Read the model definition and answer for the solid it produces. Units are mm, in the model's axes. Face numbers are marked on the shaded views. Coordinates: 2 decimals unless noted, no trailing zeros. Order: outer loops, then holes, each group sorted by start corner. A loop starts at its lowest first (then second) coordinate and runs counter-clockwise, first axis right, second up. Notation, with made-up numbers: (12, -2.5) - (69, -2.5) arc R13 ccw to (69, 21.5) - close; hole circle Ø2 at (-5.75, 83). An arc over 180 degrees is marked (long way). Write item = value, one per line.
from build123d import *

# Parameters (mm, degrees)
EXTRUDE_START       = -10
SKETCH_1_R          = 3.5
EXTRUDE_1_DEPTH     = 85
SKETCH_2_W          = 4.358557255
SKETCH_2_H          = 19.447665258
SKETCH_2_W_2        = 4.358557256
CUT_EXTRUDE_2_DEPTH = 9
SKETCH_3_R          = 1
CUT_EXTRUDE_3_DEPTH = 9


with BuildPart() as part:
    # Эскиз1 → Вытянуть1 (new body)
    with BuildSketch(Plane(origin=(0, 0, 0), x_dir=(1, 0, 0), z_dir=(0, 1, 0)).offset(EXTRUDE_START)):
        with Locations(Location((1.708090692, -2.563541488, 0), (0, 0, 270))):
            Circle(SKETCH_1_R)
    extrude(amount=EXTRUDE_1_DEPTH)

    # Эскиз2 → Вытянуть2 (cut, symmetric)
    with BuildSketch(Plane(origin=(0, 0, 0), x_dir=(0, 0, -1), z_dir=(1, 0, 0))):
        with Locations((-7.693664616, 8.043574294)):
            Rectangle(SKETCH_2_W, SKETCH_2_H)
        with Locations((2.56658164, 8.043574294)):
            Rectangle(SKETCH_2_W_2, SKETCH_2_H)
    extrude(amount=CUT_EXTRUDE_2_DEPTH, both=True, mode=Mode.SUBTRACT)

    # Эскиз3 → Вытянуть3 (cut, symmetric)
    with BuildSketch(Plane(origin=(0, 0, 0), x_dir=(0, 0, -1), z_dir=(1, 0, 0))):
        with Locations((-2.563541488, -2.980105713)):
            Circle(SKETCH_3_R)
        with Locations((-2.563541488, 8.092188022)):
            Circle(SKETCH_3_R)
    extrude(amount=CUT_EXTRUDE_3_DEPTH, both=True, mode=Mode.SUBTRACT)


solid = part.part
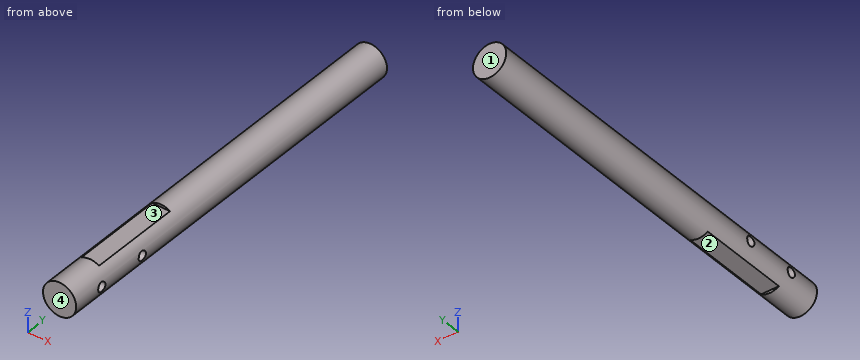
1) The part is cut by section C-C (y = 51.5). Determine the outline of the cut face in (x, z), and give its area (3 significant figures).
Returned:
outline = circle Ø7 at (1.71, 2.56)
area = 38.5 mm^2
2) The part is cut by section B-B (z = 4.5). Determine the outline of the cut face in (x, y), and give its area (3 significant figures).
Returned:
outline = (-1.21, -10) - (4.62, -10) - (4.62, 75) - (-1.21, 75) - close
area = 496 mm^2
3) Determine the mould class of the marked faces 1, 2, 3 and 4 for opening direction Y: pulls with the +Y half, pulls with the -Y half, needs draft (parallel to the pull), parting line crosses it, or undercut.
Returned:
face_1 = pulls with the +Y half
face_2 = undercut
face_3 = undercut
face_4 = pulls with the -Y half
4) Straight lines are drawn through the part: line 1 along Y through (x, z) = (1.5, 2.5); line 2 along Z through (x, y) = (1.5, 5); line 3 along Y through (x, z) = (1.5, 3). For each, find the intervals that lie inside material, in ascending order. Write a range as from..to.
Returned:
line_1 = -10..-3.98, -1.98..7.09, 9.09..75
line_2 = -0.39..5.51
line_3 = -10..-3.88, -2.08..7.19, 8.99..75
5) The part is cut by section A-A (x = 1). Determine the outline of the cut face in (y, z), and give its area (3 significant figures).
Returned:
outline = (-10, -0.86) - (-1.68, -0.86) - (-1.68, -0.39) - (17.77, -0.39) - (17.77, -0.86) - (75, -0.86) - (75, 5.99) - (17.77, 5.99) - (17.77, 5.51) - (-1.68, 5.51) - (-1.68, 5.99) - (-10, 5.99) - close; hole circle Ø2 at (-2.98, 2.56); hole circle Ø2 at (8.09, 2.56)
area = 558 mm^2
6) Flat-ended cylindrical pins translate along their axes: pin 1 Ø1 at (y, z) = (47, 3.5) entering from +X; pin 2 Ø1.5 at (y, z) = (12, 1) entering from -X; pin 3 Ø1.5 at (x, y) = (2.5, 13) entering from +Z; pin 4 Ø1.8 at (y, z) = (-2.98, 2.56) entering from +X. Find the tip coordinate at first contact, or state that the pin passes through.
Returned:
pin_1 = 5.18
pin_2 = -1.7
pin_3 = 5.51
pin_4 = through
